The figure shows three views and two pictorial views of one solid part (mm, origin at its lowest corner). Answer the questions. Give positions to 0.01 mm unless a question says otherwise; leave off trailing zeros. Order: outer loops, then holes, each group sorted by start corner. A loop starts at its lowest first (then second) coordinate and runs counter-clockwise, first axis right, second up. Notation, with made-up numbers: (78, 31) - (128, 31) arc R14 cw to (128, 46) - close; hole circle Ø6 at (-28, 27). An arc over 180 degrees is marked (long way). Write item = value, one per line.
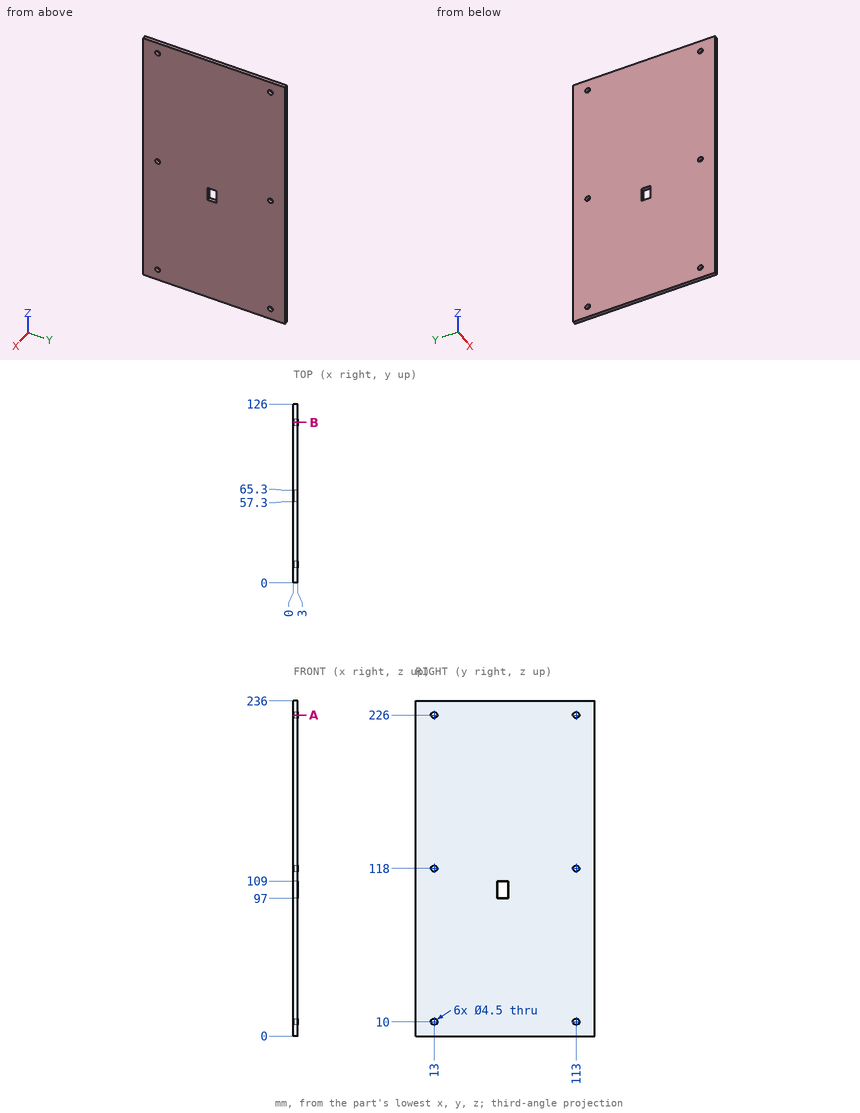
1. Section A-A (z = 226) is taken. Determine the outline of the cut face in (x, y).
Recorded:
outline = (0, 0) - (3, 0) - (3, 10.75) - (0, 10.75) - close; (0, 15.25) - (3, 15.25) - (3, 110.75) - (0, 110.75) - close; (0, 115.25) - (3, 115.25) - (3, 126) - (0, 126) - close
2. A flat-ended cylindrical pin translates along its axis: pin 1 (6 mm diameter, centred on y = 113, z = 226, fed in from +X). Find the tip coordinate at first contact, or state that the pin passes through.
Recorded:
pin_1 = 3
3. Section B-B (y = 113) is taken. Determine the outline of the cut face in (x, z), and give its area (4 significant figures).
Recorded:
outline = (0, 0) - (3, 0) - (3, 7.75) - (0, 7.75) - close; (0, 12.25) - (3, 12.25) - (3, 115.75) - (0, 115.75) - close; (0, 120.25) - (3, 120.25) - (3, 223.75) - (0, 223.75) - close; (0, 228.25) - (3, 228.25) - (3, 236) - (0, 236) - close
area = 667.5 mm^2
4. A straight line is drawn through the part: L1, parallel to Y at x = 1.15, z = 10. Find the intervals that lie inside material, in ascending order. Write a range as [from, to].
Recorded:
L1 = [0, 10.75], [15.25, 110.75], [115.25, 126]
